Design review of the part built by this model. Coordinates are the model's own, in mm. A direction names the side the tool comes from. Give positions to 0.01 mm unless a question says otherwise; leave off trailing zeros. Write each loop counter-clockwise with the first axis right and the second up, starting at its lowest first coordinate (ties: lowest second). Pieces come first, ordered by that corner, then holes. Notation, with made-up numbers: (80.5, 29) -> (90.5, 29) arc R18 cw to (90.5, 41) -> close; hole circle Ø9 at (-23, -1.75). An arc over 180 degrees is marked (long way). Put each result on its own line as item: value. Start each with the question number.
from build123d import *

# Parameters (mm, degrees)
SKETCH1_W           = 48.26
SKETCH1_H           = 25.4
BOSS_EXTRUDE1_DEPTH = 5.08
SKETCH3_W           = 5.08
SKETCH3_H           = 25.4
BOSS_EXTRUDE2_DEPTH = 31.496
SKETCH4_R           = 1.2192
CUT_EXTRUDE2_DEPTH  = 30.464
SKETCH5_W           = 25.4
SKETCH5_H           = 15.24
BOSS_EXTRUDE3_DEPTH = 16.51
SKETCH6_W           = 20.32
SKETCH6_H           = 19.05
BOSS_EXTRUDE4_DEPTH = 5.08
SKETCH7_W           = 20.32
SKETCH7_H           = 19.05
BOSS_EXTRUDE5_DEPTH = 5.08
SKETCH8_R           = 3.3782
CUT_EXTRUDE3_DEPTH  = 6.35
SKETCH9_R           = 3.3782
CUT_EXTRUDE4_DEPTH  = 6.35


with BuildPart() as part:
    # Sketch1 → Boss-Extrude1 (new body)
    with BuildSketch(Plane(origin=(0, 0, 0), x_dir=(1, 0, 0), z_dir=(0, 1, 0))):
        with Locations((24.13, 12.7)):
            Rectangle(SKETCH1_W, SKETCH1_H)
    extrude(amount=BOSS_EXTRUDE1_DEPTH)

    # Sketch3 → Boss-Extrude2 (add)
    with BuildSketch(Plane(origin=(0, 5.08, 0), x_dir=(1, 0, 0), z_dir=(0, 1, 0))):
        with Locations((26.924, 12.7)):
            Rectangle(SKETCH3_W, SKETCH3_H)
        with Locations((15.494, 12.7)):
            Rectangle(SKETCH3_W, SKETCH3_H)
    extrude(amount=BOSS_EXTRUDE2_DEPTH)

    # Sketch4 → Cut-Extrude2 (cut, through all)
    with BuildSketch(Plane(origin=(29.464, 0, 0), x_dir=(0, 0, -1), z_dir=(1, 0, 0))):
        with Locations((12.7, 34.036)):
            Circle(SKETCH4_R)
    extrude(amount=-CUT_EXTRUDE2_DEPTH, mode=Mode.SUBTRACT)

    # Sketch5 → Boss-Extrude3 (add)
    with BuildSketch(Plane(origin=(29.464, 0, 0), x_dir=(0, 0, -1), z_dir=(1, 0, 0))):
        with Locations((12.7, 12.7)):
            Rectangle(SKETCH5_W, SKETCH5_H)
    extrude(amount=-BOSS_EXTRUDE3_DEPTH)

    # Sketch6 → Boss-Extrude4 (add)
    with BuildSketch(Plane.ZY):
        with Locations((-12.7, -4.445)):
            Rectangle(SKETCH6_W, SKETCH6_H)
    extrude(amount=BOSS_EXTRUDE4_DEPTH)

    # Sketch7 → Boss-Extrude5 (add)
    with BuildSketch(Plane(origin=(48.26, 0, 0), x_dir=(0, 0, -1), z_dir=(1, 0, 0))):
        with Locations((12.7, -4.445)):
            Rectangle(SKETCH7_W, SKETCH7_H)
    extrude(amount=BOSS_EXTRUDE5_DEPTH)

    # Sketch8 → Cut-Extrude3 (cut)
    with BuildSketch(Plane(origin=(53.34, 0, 0), x_dir=(0, 0, -1), z_dir=(1, 0, 0))):
        with Locations((12.7, -6.35)):
            Circle(SKETCH8_R)
    extrude(amount=-CUT_EXTRUDE3_DEPTH, mode=Mode.SUBTRACT)

    # Sketch9 → Cut-Extrude4 (cut)
    with BuildSketch(Plane.ZY.offset(5.08)):
        with Locations((-12.7, -6.35)):
            Circle(SKETCH9_R)
    extrude(amount=-CUT_EXTRUDE4_DEPTH, mode=Mode.SUBTRACT)


solid = part.part
Q1. Machinability: for faces 4 (the face through (24, 0, -13)), 5 (the face through (12.954, 21, -13)), 6 (the face through (51, -5, -22.86)), 7 (the face through (-3, -5, -2.54)), 8 (the face through (0, 3, -24)), which of the approach directions +Z, -Z, +X, -X, +Y, -Y give a long, thin tool a straight path to every point of the face, cutting with its end or side? Answer none if there is none.
Q2. To check wall thickness, follow probe 1 along Y at (x, z) = (-1.8, -12.7); probe 2 along X at (y, z) = (-10, -19); probe 3 along Y at (x, z) = (15.35, -12.7). State the ranges of each line that lie inside material, in increasing order. Write a range as from..to.
Q3. Mouldability with a two-part tool opening along X and no side actions: class faces 1 (the face through (18.034, 28, -13)), 2 (the face through (48.26, 3, -24)), 3 (the face through (-3, -5, -22.86)) as +X half, -X half, draft (parallel to the pull), parting line (faces both ways), or undercut.
Q4. Take a section at A-A on z = -12.7. State how many separate pieces and enclosed holes the cut face has, then the cut area to 3 significant figures.
Q5. Take a section at D-D on y = 2.5. Give the boundary of the cut face in (x, z).
Q6. For pin 1 (7.5 mm diameter, centred on y = 15, z = -7, fed in from +X); pin 2 (3 mm diameter, centred on x = 16.5, z = -8, fed in from -Y); pin 3 (2.5 mm diameter, centred on x = 52, y = -7, fed in from -Z), all flat-tipped, find the tip position at first contact; note any pin that passes through.
Q7. Take a section at B-B on y = -6.35. Give the boundary of the cut face in (x, z).
Q8. Take a section at C-C on z = -17.75. Give the boundary of the cut face in (x, y).
Result:
1. face 4: +Z, -Z, -Y
1. face 5: +Z, -Z, -X, +Y
1. face 6: -Z, +X, +Y, -Y
1. face 7: +Z, -X, +Y, -Y
1. face 8: -Z, -X, +Y, -Y
2. probe 1: y = -13.97..-9.73, -2.97..5.08
2. probe 2: x = -5.08..0, 48.26..53.34
2. probe 3: y = 0..32.82, 35.26..36.58
3. face 1: undercut
3. face 2: +X half
3. face 3: draft
4. separate pieces: 5
4. enclosed holes: 0
4. area: 762 mm^2
5. outline: (-5.08, -22.86) -> (0, -22.86) -> (0, -25.4) -> (48.26, -25.4) -> (48.26, -22.86) -> (53.34, -22.86) -> (53.34, -2.54) -> (48.26, -2.54) -> (48.26, 0) -> (0, 0) -> (0, -2.54) -> (-5.08, -2.54) -> close
6. pin 1: stops at x = 29.46
6. pin 2: stops at y = 0
6. pin 3: stops at z = -22.86
7. outline: (-5.08, -22.86) -> (0, -22.86) -> (0, -16.08) -> (-5.08, -16.08) -> close; (-5.08, -9.32) -> (0, -9.32) -> (0, -2.54) -> (-5.08, -2.54) -> close; (48.26, -22.86) -> (53.34, -22.86) -> (53.34, -16.08) -> (48.26, -16.08) -> close; (48.26, -9.32) -> (53.34, -9.32) -> (53.34, -2.54) -> (48.26, -2.54) -> close
8. outline: (-5.08, -13.97) -> (0, -13.97) -> (0, 0) -> (48.26, 0) -> (48.26, -13.97) -> (53.34, -13.97) -> (53.34, 5.08) -> (29.46, 5.08) -> (29.46, 36.58) -> (24.38, 36.58) -> (24.38, 20.32) -> (18.03, 20.32) -> (18.03, 36.58) -> (12.95, 36.58) -> (12.95, 5.08) -> (-5.08, 5.08) -> close
